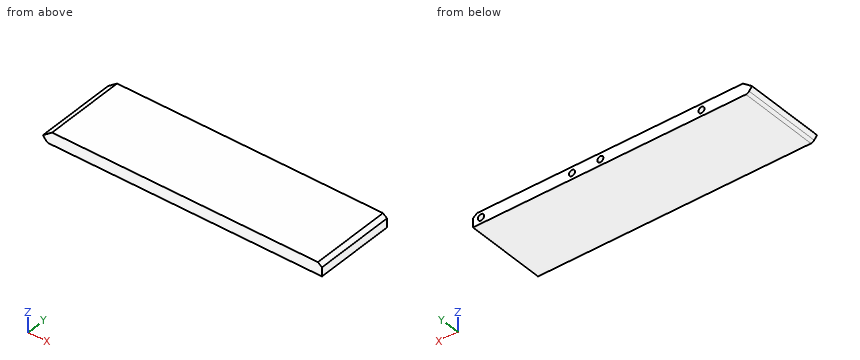
```python
from build123d import *

# Parameters (mm, degrees)
BOSS_EXTRUDE1_DEPTH     = 20
SKETCH2_R               = 1.5
SKETCH2_R_2             = 1.572515875
CUT_EXTRUDE1_DEPTH      = 5
FILLET1_R               = 2
SKETCH3_W               = 103.784472799
SKETCH3_H               = 73.748761466
CUT_EXTRUDE2_DEPTH      = 184.826439883
CUT_EXTRUDE3_DEPTH      = 85.597401851
CUT_EXTRUDE3_DEPTH_BACK = 85.597401851
SKETCH4_W               = 26
SKETCH4_H               = 40
CUT_EXTRUDE4_DEPTH      = 100.602813213
CUT_EXTRUDE4_DEPTH_BACK = 100.602813213


with BuildPart() as part:
    # Sketch1 → Boss-Extrude1 (new, symmetric)
    with BuildSketch(Plane(origin=(0, 0, 0), x_dir=(1, 0, 0), z_dir=(0, 1, 0))):
        Polygon((-110, 0), (-80, 40), (80, 40), (110, 0), (103, 0), (77.5, 34), (-77.5, 34), (-103, 0), align=None)
    extrude(amount=BOSS_EXTRUDE1_DEPTH, both=True)

    # Sketch2 → Cut-Extrude1 (cut)
    with BuildSketch(Plane(origin=(0, 20, 0), x_dir=(1, 0, 0), z_dir=(0, 1, 0))):
        with Locations(Location((-104, 3, 0), (0, 0, 270))):
            Circle(SKETCH2_R)
        with Locations(Location((-57, 37, 0), (0, 0, 270))):
            Circle(SKETCH2_R)
        with Locations(Location((-7, 37, 0), (0, 0, 270))):
            Circle(SKETCH2_R)
        with Locations(Location((7, 37, 0), (0, 0, 90))):
            Circle(SKETCH2_R)
        with Locations(Location((104, 3, 0), (0, 0, 90))):
            Circle(SKETCH2_R)
        with Locations(Location((52, 37, 0), (0, 0, 270))):
            Circle(SKETCH2_R_2)
    extrude(amount=-CUT_EXTRUDE1_DEPTH, mode=Mode.SUBTRACT)

    # Fillet1
    fillet1_edges = [part.edges().sort_by_distance(p)[0] for p in [
        (-80, 0, -40),
        (80, 0, -40),
    ]]
    fillet(fillet1_edges, radius=FILLET1_R)

    # Sketch3 → Cut-Extrude2 (cut, symmetric)
    with BuildSketch(Plane(origin=(-65.92, 0, -49.44), x_dir=(0.5999999999999999, 0, -0.8000000000000002), z_dir=(0.8000000000000003, 0, 0.5999999999999999))):
        with Locations((-71.1922364, 16.874380733)):
            Rectangle(SKETCH3_W, SKETCH3_H)
    cut_extrude2 = extrude(amount=CUT_EXTRUDE2_DEPTH, both=True, mode=Mode.SUBTRACT)

    # Mirror1: Cut-Extrude2 across plane
    add(cut_extrude2.mirror(Plane(origin=(0, 0, 0), x_dir=(0, 0, 1), z_dir=(1, 0, 0))), mode=Mode.SUBTRACT)

    # Sketch4 → Cut-Extrude3 (cut, two sides: drawn at the far end of the back side and taken through both)
    with BuildSketch(Plane.XY.offset(-34).offset(-CUT_EXTRUDE3_DEPTH_BACK)):
        with Locations((68.98, 0)):
            Rectangle(SKETCH4_W, SKETCH4_H)
    extrude(amount=CUT_EXTRUDE3_DEPTH + CUT_EXTRUDE3_DEPTH_BACK, mode=Mode.SUBTRACT)

    # Sketch5 → Cut-Extrude4 (cut, two sides: drawn at the far end of the back side and taken through both)
    with BuildSketch(Plane.XZ.offset(20).offset(-CUT_EXTRUDE4_DEPTH_BACK)):
        Polygon((55.98, -35.588024178), (53.98, -34), (55.98, -34), align=None)
    extrude(amount=CUT_EXTRUDE4_DEPTH + CUT_EXTRUDE4_DEPTH_BACK, mode=Mode.SUBTRACT)


solid = part.part
```
Geometry: final body of the model. Coordinates: model frame, mm. Give positions to 0.01 mm unless a question says otherwise; leave off trailing zeros. Write each loop counter-clockwise with the first axis right and the second up, starting at its lowest first coordinate (ties: lowest second). Pieces come first, ordered by that corner, then holes.
1. Section query B-B, the plane x = 52. Return loops of the section in (y, z), then the cut area to 3 significant figures.
2. Pin query (flat end, axial travel): P1, Ø0.9, axis at x = -57, z = -37, coming from the +Y side. Return the tip coordinate at first contact, or that it passes through.
3. Section query A-A, the plane x = -7. Return loops of the section in (y, z), then the cut area to 3 significant figures.
4. Line query: probe 1 along Z at (x, y) = (7, 18.75); probe 2 along X at (y, z) = (17.75, -37); probe 3 along X at (y, z) = (-5, -37.75). Output: solid intervals per line, ascending.
Computed:
1. outline: (-20, -40) - (20, -40) - (20, -38.57) - (15, -38.57) - (15, -35.43) - (20, -35.43) - (20, -34) - (-20, -34) - close
1. area: 224 mm2
2. P1: stops at y = 15
3. outline: (-20, -40) - (20, -40) - (20, -38.5) - (15, -38.5) - (15, -35.5) - (20, -35.5) - (20, -34) - (-20, -34) - close
3. area: 225 mm2
4. probe 1: z = -40 to -38.5, -35.5 to -34
4. probe 2: x = -81.5 to -58.5, -55.5 to -8.5, -5.5 to 5.5, 8.5 to 50.43, 53.57 to 55.98
4. probe 3: x = -81.69 to 55.98
